from build123d import *

# Parameters (mm, degrees)
SKETCH_1_W             = 41
SKETCH_1_H             = 15.5
SM_BASE_FLANGE_1_DEPTH = 1
SKETCH_6_W             = 6
SKETCH_6_H             = 6
EXTRUDE_1_DEPTH        = 10
SKETCH_7_R             = 2.75
EXTRUDE_2_DEPTH        = 4
SKETCH_8_R             = 5
EXTRUDE_3_DEPTH        = 30
SKETCH_9_R             = 5
EXTRUDE_4_DEPTH        = 87
FILLET_1_R             = 4
SKETCH_10_W            = 6
SKETCH_10_H            = 10
EXTRUDE_5_DEPTH        = 15


# Sheet-metal steps are written as plain solids
with BuildPart() as part:
    # Sketch 1 → Базовая кромка1 (new body)
    with BuildSketch(Plane(origin=(0, 0, 0), x_dir=(1, 0, 0), z_dir=(0, 1, 0))):
        Rectangle(SKETCH_1_W, SKETCH_1_H)
    extrude(amount=-SM_BASE_FLANGE_1_DEPTH)

    # Эскиз6 → Бобышка-Вытянуть1 (add)
    with BuildSketch(Plane(origin=(0, 0, 0), x_dir=(1, 0, 0), z_dir=(0, 1, 0))):
        with Locations((17.5, 0)):
            Rectangle(SKETCH_6_W, SKETCH_6_H)
    extrude(amount=EXTRUDE_1_DEPTH)

    # Эскиз7 → Бобышка-Вытянуть2 (add)
    with BuildSketch(Plane(origin=(20.5, 0, 0), x_dir=(0, 0, -1), z_dir=(1, 0, 0))):
        with Locations((0, 7)):
            Circle(SKETCH_7_R)
    extrude(amount=EXTRUDE_2_DEPTH)

    # Эскиз8 → Бобышка-Вытянуть3 (add)
    with BuildSketch(Plane(origin=(24.5, 0, 0), x_dir=(0, 0, -1), z_dir=(1, 0, 0))):
        with Locations((0, 7)):
            Circle(SKETCH_8_R)
    extrude(amount=EXTRUDE_3_DEPTH)

    # Эскиз9 → Бобышка-Вытянуть4 (add)
    with BuildSketch(Plane(origin=(0, 2, 0), x_dir=(-1, 0, 0), z_dir=(0, -1, 0))):
        with Locations(Location((-49.5, 0, 0), (0, 0, 90))):
            Circle(SKETCH_9_R)
    extrude(amount=-EXTRUDE_4_DEPTH)

    # Скругление1
    fillet_1_edges = [part.edges().sort_by_distance(p)[0] for p in [
        (49.5, 89, 5),
    ]]
    fillet(fillet_1_edges, radius=FILLET_1_R)

    # Эскиз10 → Бобышка-Вытянуть5 (add)
    with BuildSketch(Plane.XZ.offset(1)):
        with Locations((-17.5, 0)):
            Rectangle(SKETCH_10_W, SKETCH_10_H)
    extrude(amount=EXTRUDE_5_DEPTH)


solid = part.part
Here's how the part is built. I have some questions about the finished solid (model axes, mm). A direction names the side the tool comes from. Coordinates: 2 decimals unless noted, no trailing zeros. Write each loop counter-clockwise with the first axis right and the second up, starting at its lowest first coordinate (ties: lowest second). Pieces come first, ordered by that corner, then holes.
Item 1: If I drill on line 1 (Y direction, x = 18, z = -3.5); line 2 (X direction, y = 11, z = 2.5); line 3 (X direction, y = -10.5, z = 3.75), over which ranges is the centre line in solid material (lowest first)?
Item 2: If we mould it in two halves opening along X, with no side actions, what happens to faces 1 (the flat face through (-18, -8, -5)), 2 (the flat face through (54.5, 7, 0)), 3 (the flat face through (24.5, 4.8, -2.2))? For each: +X half, -X half, draft (parallel to the pull), parting line (faces both ways), or undercut.
Item 3: I want a section at C-C on y = 17. Write out the boundary of the cut face in (x, z), and give its area (3 significant figures).
Item 4: Will these pins go through, and if not, where does the flat tip stop? pin 1 (8 mm diameter, centred on y = 32, z = 4.5, fed in from +X); pin 2 (5 mm diameter, centred on y = 5, z = 0.5, fed in from -X); pin 3 (1.8 mm diameter, centred on x = -18, y = -9.5, fed in from +Z).
Item 5: I want a section at D-D on x = 36.5. Write out the boundary of the cut face in (y, z).
Item 6: I want a section at A-A on x = 6. Write out the boundary of the cut face in (y, z).
Item 7: On a 3-axis mill with a long thin cutter (end or side, diameter ignored), from which of +Z, -Z, +X, -X, +Y, -Y can I reach the whole of each face in a straight line? I mean faces 4 (the cylindrical face through (49.72, 45.454, 4.995)), 5 (the cylindrical face through (53, 7, 5)), 6 (the cylindrical face through (53, 7, -5)), 7 (the flat face through (17, 5, -3)). Say none if no direction works.
Item 8: I want a section at B-B on z = 6.25. Write out the boundary of the cut face in (x, y).
Findings below:
1. line 1: y = -1 to 0
1. line 2: x = 24.5 to 54.5
1. line 3: x = -20.5 to -14.5
2. face 1: draft
2. face 2: +X half
2. face 3: undercut
3. outline: circle Ø10 at (49.5, 0)
3. area: 78.5 mm2
4. pin 1: stops at x = 54.47
4. pin 2: stops at x = 14.5
4. pin 3: stops at z = 5
5. outline: circle Ø10 at (7, 0)
6. outline: (-1, -7.75) - (0, -7.75) - (0, 7.75) - (-1, 7.75) - close
7. face 4: +Y
7. face 5: +Z, +X
7. face 6: -Z, +X
7. face 7: -Z, -X, +Y
8. outline: (-20.5, -1) - (20.5, -1) - (20.5, 0) - (-20.5, 0) - close
